```python
from build123d import *

# Parameters (mm, degrees)
CHAMFER1_SIZE      = 0.875
CUT_EXTRUDE1_START = -6.000000232
CUT_EXTRUDE1_DEPTH = 6.000000232
FILLET2_R          = 0.6


with BuildPart() as part:
    # Sketch1 → Revolve1 (revolve)
    with BuildSketch(Plane(origin=(0, 0, 0), x_dir=(0, 0, -1), z_dir=(1, 0, 0)), mode=Mode.PRIVATE) as revolve1_sk:
        Polygon((0, 10), (-12, 10), (-12, 0), (200, 0), (200, 7), (0, 7), align=None)
    revolve(revolve1_sk.sketch.rotate(Axis((0, 0, 12), (0, 0, -1)), 180), axis=Axis((0, 0, 12), (0, 0, -1)))

    # Sketch7 → Cut-Revolve2 (revolve, cut)
    with BuildSketch(Plane(origin=(0, 0, 0), x_dir=(0, 0, -1), z_dir=(1, 0, 0)), mode=Mode.PRIVATE) as cut_revolve2_sk:
        Polygon((-12, 0), (-12, 5), (-6, 5), (-3.113248654, 0), align=None)
    revolve(cut_revolve2_sk.sketch.rotate(Axis((0, 0, 12), (0, 0, -1)), 90), axis=Axis((0, 0, 12), (0, 0, -1)), mode=Mode.SUBTRACT)

    # Chamfer1
    chamfer1_edges = [part.edges().sort_by_distance(p)[0] for p in [
        (0, 10, 12),
        (0, 7, -200),
    ]]
    chamfer(chamfer1_edges, length=CHAMFER1_SIZE)

    # Cut-Extrude1: read off the stored shape, not the designer's step
    # Cut-Extrude1 outline → Cut-Extrude1 (cut)
    with BuildSketch(Plane.XY.offset(12).offset(CUT_EXTRUDE1_START)):
        with BuildLine():
            Line((5, 0), (5, 2.886751346))
            Line((5, 2.886751346), (2.500000011, 4.330127013))
            ThreePointArc((2.500000011, 4.330127013), (4.330127022, 2.499999995), (5, 0))
        make_face()
        with BuildLine():
            ThreePointArc((-2.500000011, 4.330127013), (0, 5), (2.500000011, 4.330127013))
            Line((2.500000011, 4.330127013), (0, 5.773502692))
            Line((0, 5.773502692), (-2.500000011, 4.330127013))
        make_face()
        with BuildLine():
            Line((5, -2.886751346), (5, 0))
            ThreePointArc((5, 0), (4.330127007, -2.500000021), (2.499999959, -4.330127043))
            Line((2.499999959, -4.330127043), (5, -2.886751346))
        make_face()
        with BuildLine():
            ThreePointArc((-5, 0), (-4.330127022, 2.499999995), (-2.500000011, 4.330127013))
            Line((-2.500000011, 4.330127013), (-5, 2.886751346))
            Line((-5, 2.886751346), (-5, 0))
        make_face()
        with BuildLine():
            Line((0, -5.773502692), (2.499999959, -4.330127043))
            ThreePointArc((2.499999959, -4.330127043), (-6e-08, -5), (-2.500000063, -4.330126983))
            Line((-2.500000063, -4.330126983), (0, -5.773502692))
        make_face()
        with BuildLine():
            ThreePointArc((-2.500000063, -4.330126983), (-4.330127037, -2.499999969), (-5, 0))
            Line((-5, 0), (-5, -2.886751346))
            Line((-5, -2.886751346), (-2.500000063, -4.330126983))
        make_face()
    extrude(amount=CUT_EXTRUDE1_DEPTH, mode=Mode.SUBTRACT)

    # Cut-Extrude1 2 outline → Cut-Extrude1 2 (revolve)
    with BuildSketch(Plane.XZ):
        Polygon((5.773502705, 6.446581995), (4.9999999, 5.999999942), (5.773502692, 5.999999768), align=None)
    revolve(axis=Axis((0, 0, 0), (0, 0, 1)))

    # Sketch9 → Cut-Revolve3 (revolve, cut)
    with BuildSketch(Plane(origin=(0, 0, 0), x_dir=(0, 0, -1), z_dir=(1, 0, 0))):
        Polygon((-12.5, 6.639528096), (-12.5, 5), (-11.553418013, 5), align=None)
    revolve(axis=Axis((0, 0, 12), (0, 0, -1)), mode=Mode.SUBTRACT)

    # Fillet2
    fillet2_edges = [part.edges().sort_by_distance(p)[0] for p in [
        (0, 7, 0),
    ]]
    fillet(fillet2_edges, radius=FILLET2_R)


solid = part.part
```
Geometry check sheet. Reference: the model listing, model coordinates, mm. A direction names the side the tool comes from. Give positions to 0.01 mm unless a question says otherwise; leave off trailing zeros. Write each loop counter-clockwise with the first axis right and the second up, starting at its lowest first coordinate (ties: lowest second). Pieces come first, ordered by that corner, then holes. Notation, with made-up numbers: (7, 7) -> (56, 7) arc R18 ccw to (56, 13) -> close; hole circle Ø1 at (-4, 7.25). An arc over 180 degrees is marked (long way). One line per question, with ' | ' between items.
Item 1: Depth check by flat-ended pin: pin 1 (4 mm diameter, centred on x = 4, z = -173.5, fed in from -Y); pin 2 (5 mm diameter, centred on y = -1.5, z = -55.5, fed in from +X); pin 3 (8 mm diameter, centred on y = 6.5, z = -175.5, fed in from -X). Enter the tip coordinate at first touch or a pass-through.
Determined:
pin 1: y = -6.71 | pin 2: x = 7 | pin 3: x = -6.54
Item 2: Scan lines: line 1 along Y through (x, z) = (-0.75, -103.5); line 2 along X through (y, z) = (0.25, -169); line 3 along Z through (x, y) = (3, -8.25). Record each from-to range of solid material in increasing order.
Determined:
line 1: -6.96 to 6.96 | line 2: -7 to 7 | line 3: 0 to 12
Item 3: Draft check along Y on faces 4 (the cylindrical face through (2.681, -6.466, -98.473)), 5 (the flat face through (5, 0, 9)), 6 (the flat face through (6, 0, 12)). Enter one of: released by +Y, released by -Y, zero draft, split by the parting line, or undercut.
Determined:
face 4: split by the parting line | face 5: undercut | face 6: zero draft
Item 4: Sectioned sample at A-A, the plane z = -10. Record the boundary of the cut face in (x, y), plus the area to 3 significant figures.
Determined:
outline: circle Ø14 at (0, 0) | area: 154 mm^2
Item 5: Access from +Z, -Z, +X, -X, +Y, -Y to the whole of each face (thin tool, end or side, straight path). Record for faces 1 (the flat face through (-4, 7, 0)), 2 (the flat face through (0, 0, -200)), 3 (the flat face through (-5, 0, 9)).
Determined:
face 1: -Z | face 2: -Z, +X, -X, +Y, -Y | face 3: +Z
